Verification items for the finished model (mm, model axes). A direction names the side the tool comes from. Round coordinates to 2 decimals unless told otherwise and drop trailing zeros. Order: outer loops, then holes, each group sorted by start corner. A loop starts at its lowest first (then second) coordinate and runs counter-clockwise, first axis right, second up. Notation, with made-up numbers: M 78,84.25 L 97,84.25 A14 cw 97,108.25 Z; hole C 43.25,13.5 d4. An arc over 180 degrees is marked long. Use CSV: the item, a comma, the result in double quotes. Start each with the question number.
Q1. Mould release check, pull along Z, two halves, no side actions. Record for faces 3 (the face through (0, -39.3, 21.3)), 4 (the face through (14.168, -25.861, -33.727)), 5 (the face through (25.884, -33.497, -43.686)): +Z half, -Z half, draft (parallel to the pull), parting line (faces both ways), or undercut.
Q2. Sectioned sample at A-A (y = 0). Enter the section's corners in (x, z), and give its area (3 significant figures).
Q3. Sectioned sample at C-C (x = 4.5). Enter the section's corners in (y, z), and give its area (3 significant figures).
Q4. Gauge pin test, flat ends, axial feed: pin 1 Ø10 at (x, y) = (5, -7.5) entering from +Z; pin 2 Ø2 at (x, z) = (11, -14) entering from -Y; pin 3 Ø2 at (x, z) = (9.5, -17) entering from -Y. Record the tip position at first contact, or that the pin passes through.
Q5. Sectioned sample at D-D (x = 15). Enter the section's corners in (y, z).
Q6. Scan lines: line 1 (Y direction, x = 9.75, z = 0); line 2 (Z direction, x = 10, y = 33.5); line 3 (Z direction, x = 22.5, y = -35). Record each from-to range of solid material in increasing order.
Q7. Set-up check for faces 1 (the face through (5.76, 32.79, -35.75)), 2 (the face through (28, 0, -45)): record each of +Z, -Z, +X, -X, +Y, -Y from which the full face is reachable in a straight line by a thin tool's end or side.
```python
from build123d import *


with BuildPart() as part:
    # Schizzo1 → Rivoluzione1 (revolve)
    with BuildSketch(Plane.XY, mode=Mode.PRIVATE) as rivoluzione1_sk:
        with BuildLine():
            Line((0, 48.51), (0, 44.5))
            ThreePointArc((0, 44.5), (0.585786438, 43.085786438), (2, 42.5))
            Line((2, 42.5), (26, 42.5))
            ThreePointArc((26, 42.5), (27.414213562, 43.085786438), (28, 44.5))
            Line((28, 44.5), (28, 55.05))
            Line((28, 55.05), (23.826494797, 55.05))
            ThreePointArc((23.826494797, 55.05), (18.977115837, 49.504551501), (11.677845828, 48.51))
            Line((11.677845828, 48.51), (0, 48.51))
        make_face()
    revolve(rivoluzione1_sk.sketch.rotate(Axis((28, 0, 0), (-1, 0, 0)), 270), axis=Axis((28, 0, 0), (-1, 0, 0)))


solid = part.part
```
Verdict:
1,face 3,"draft"
1,face 4,"undercut"
1,face 5,"parting line"
2,outline,"M 0,-48.51 L 11.68,-48.51 A10.5 cw 23.83,-55.05 L 28,-55.05 L 28,-44.5 A2 ccw 26,-42.5 L 2,-42.5 A2 ccw 0,-44.5 Z; M 0,44.5 A2 ccw 2,42.5 L 26,42.5 A2 ccw 28,44.5 L 28,55.05 L 23.83,55.05 A10.5 cw 11.68,48.51 L 0,48.51 Z"
2,area,"418 mm²"
3,outline,"C 0,0 d97.02; hole C 0,0 d85"
3,area,"1,720 mm²"
4,pin 1,"stops at z = 48.45"
4,pin 2,"stops at y = -46.74"
4,pin 3,"stops at y = -45.8"
5,outline,"C 0,0 d96.6; hole C 0,0 d85"
6,line 1,"y = -48.51 to -42.5, 42.5 to 48.51"
6,line 2,"z = -35.09 to -26.15, 26.15 to 35.09"
6,line 3,"z = -39.25 to -24.11, 24.11 to 39.25"
7,face 1,"-X"
7,face 2,"+Z, -Z, +X, +Y, -Y"
